Work out the finished part from the listing and answer in its coordinate system (mm). A direction names the side the tool comes from. Coordinates: 2 decimals unless noted, no trailing zeros. Order: outer loops, then holes, each group sorted by start corner. A loop starts at its lowest first (then second) coordinate and runs counter-clockwise, first axis right, second up. Notation, with made-up numbers: (28, 54) -> (39, 54) arc R26 cw to (39, 75) -> close; hole circle Ø6 at (-24.75, 54). An arc over 180 degrees is marked (long way). Use one line per item in the form item = value.
from build123d import *

# Parameters (mm, degrees)
SKETCH_1_R               = 12.5
SKETCH_1_R_2             = 7.5
EXTRUDE_1_DEPTH          = 3.95
SKETCH_2_R               = 14
SKETCH_2_R_2             = 7.5
EXTRUDE_2_DEPTH          = 1.2
HOLE_WIZARD_M2_5_1_D     = 2.05
PATTERN_CIRCULAR_1_COUNT = 4


with BuildPart() as part:
    # 草图1 → 凸台-拉伸1 (new body)
    with BuildSketch(Plane.XY):
        Circle(SKETCH_1_R)
        Circle(SKETCH_1_R_2, mode=Mode.SUBTRACT)
    extrude(amount=EXTRUDE_1_DEPTH)

    # 草图2 → 凸台-拉伸2 (add)
    with BuildSketch(Plane.XY.offset(3.95)):
        Circle(SKETCH_2_R)
        Circle(SKETCH_2_R_2, mode=Mode.SUBTRACT)
    extrude(amount=EXTRUDE_2_DEPTH)

    # M2.5 螺纹孔1 (through all)
    with Locations(Plane(origin=(0, 0, 0), x_dir=(-1, 0, 0), z_dir=(0, 0, -1))):
        with Locations((0, 10)):
            hole_wizard_m2_5_1 = Hole(HOLE_WIZARD_M2_5_1_D / 2)

    # 阵列(圆周)1: M2.5 螺纹孔1 ×4 about axis
    pattern_circular_1_axis = Axis((0, 0, 0), (0, 0, 1))
    for i in range(1, PATTERN_CIRCULAR_1_COUNT):
        add(hole_wizard_m2_5_1.rotate(pattern_circular_1_axis, i * 360 / PATTERN_CIRCULAR_1_COUNT), mode=Mode.SUBTRACT)


solid = part.part
(1) Section D-D on x = 0 is taken. Write down the section's boundary in (y, z) (3 decimals).
Data:
outline = (-14, 3.95) -> (-12.5, 3.95) -> (-12.5, 0) -> (-11.025, 0) -> (-11.025, 5.15) -> (-14, 5.15) -> close; (-8.975, 0) -> (-7.5, 0) -> (-7.5, 5.15) -> (-8.975, 5.15) -> close; (7.5, 0) -> (8.975, 0) -> (8.975, 5.15) -> (7.5, 5.15) -> close; (11.025, 0) -> (12.5, 0) -> (12.5, 3.95) -> (14, 3.95) -> (14, 5.15) -> (11.025, 5.15) -> close
(2) Section A-A on x = -4 is taken. Write down the section's boundary in (y, z).
Data:
outline = (-13.42, 3.95) -> (-11.84, 3.95) -> (-11.84, 0) -> (-6.34, 0) -> (-6.34, 5.15) -> (-13.42, 5.15) -> close; (6.34, 0) -> (11.84, 0) -> (11.84, 3.95) -> (13.42, 3.95) -> (13.42, 5.15) -> (6.34, 5.15) -> close
(3) Section B-B on y = 2.25 is taken. Write down the section's boundary in (x, z).
Data:
outline = (-13.82, 3.95) -> (-12.3, 3.95) -> (-12.3, 0) -> (-7.15, 0) -> (-7.15, 5.15) -> (-13.82, 5.15) -> close; (7.15, 0) -> (12.3, 0) -> (12.3, 3.95) -> (13.82, 3.95) -> (13.82, 5.15) -> (7.15, 5.15) -> close
(4) The mould has two halves that part along X. Classify faces 3 (the flat face through (-5.3, 11.5, 3.95)), 4 (the cylindrical face through (-7.493, 0.33, 2.539)), 5 (the cylindrical face through (12.932, -5.362, 4.542)): released by +X, released by -X, zero draft, split by the parting line, or undercut.
Data:
face_3 = zero draft
face_4 = undercut
face_5 = split by the parting line
(5) Which of the six approach directions +Z, -Z, +X, -X, +Y, -Y give full straight-line access (tool end or side, diameter ignored) to faces 1 (the flat face through (6, -6, 5.15)), 2 (the cylindrical face through (11.923, 3.755, 1.947))?
Data:
face_1 = +Z, +X, -X, +Y, -Y
face_2 = -Z
(6) Section C-C on z = 1.55 is taken. Write down the section's boundary in (x, y) (3 decimals), plus the area to 3 significant figures.
Data:
outline = circle Ø25 at (0, 0); hole circle Ø2.05 at (-10, 0); hole circle Ø15 at (0, 0); hole circle Ø2.05 at (0, -10); hole circle Ø2.05 at (0, 10); hole circle Ø2.05 at (10, 0)
area = 301 mm²
(7) Straight lines are drawn through the part: line 1 along Y through (x, z) = (0, 1.25) (3 decimals); line 2 along Y through (x, z) = (0, 4.1) (3 decimals); line 3 along Y through (x, z) = (-10, 1.55) (3 decimals). For each, find the intervals that lie inside material, in ascending order.
Data:
line_1 = -12.5 to -11.025, -8.975 to -7.5, 7.5 to 8.975, 11.025 to 12.5
line_2 = -14 to -11.025, -8.975 to -7.5, 7.5 to 8.975, 11.025 to 14
line_3 = -7.5 to -1.025, 1.025 to 7.5
(8) Each of these flat-tipped pins is pushed along its axis until it touches: P1, Ø2, axis at y = -5, z = 1.5, coming from the -X side; P2, Ø1.5, axis at x = -8, y = -11, coming from the -Z side; P3, Ø1.5, axis at y = 8, z = 3, coming from the -X side; P4, Ø1.2, axis at x = 0, y = -10, coming from the -Z side. Where does it stop, or does it pass through?
Data:
P1 = -11.84
P2 = 3.95
P3 = -10.18
P4 = through
